Input: dimensioned drawing with shaded views. Units: mm. Origin: part minimum x, y, z. A direction names the side the tool comes from. Coordinates: 2 decimals unless noted, no trailing zeros. Write each loop counter-clockwise with the first axis right and the second up, starting at its lowest first coordinate (ties: lowest second). Pieces come first, ordered by that corner, then holes. Notation, with made-up numbers: (63, -21.75) - (114, -21.75) arc R12 ccw to (114, -8.75) - close; hole circle Ø5 at (22, 84). An arc over 180 degrees is marked (long way). One line per question, with ' | ' between items.
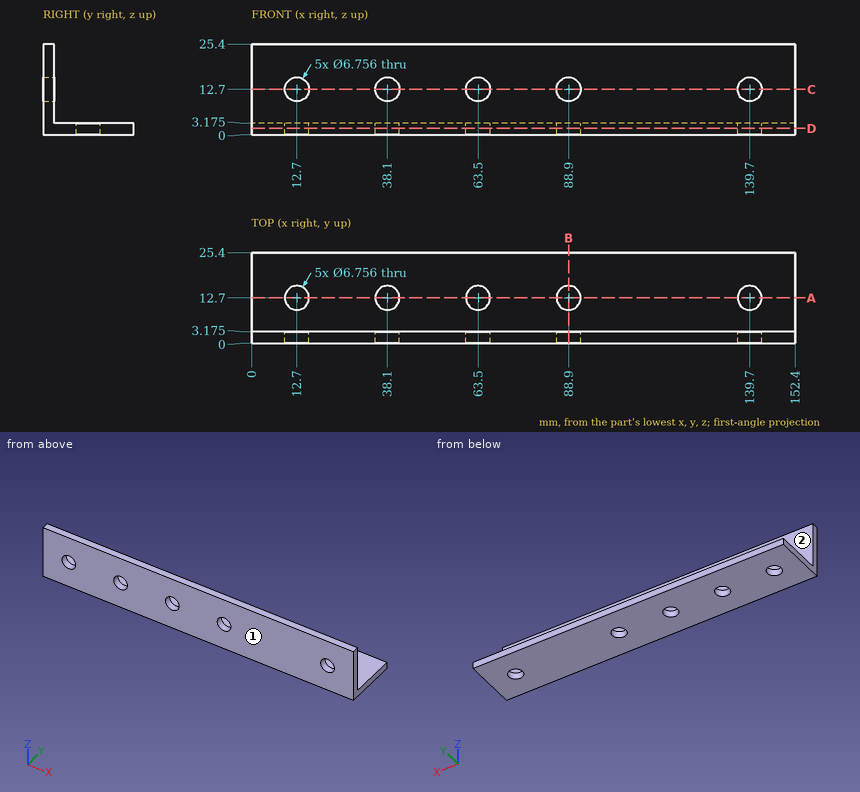
Item 1: Cut plane D-D on z = 1.75. Return loops of the section in (x, y).
Check sheet entries:
outline: (0, 0) - (152.4, 0) - (152.4, 25.4) - (0, 25.4) - close; hole circle Ø6.76 at (12.7, 12.7); hole circle Ø6.76 at (38.1, 12.7); hole circle Ø6.76 at (63.5, 12.7); hole circle Ø6.76 at (88.9, 12.7); hole circle Ø6.76 at (139.7, 12.7)
Item 2: Cut plane B-B on x = 88.9. Return loops of the section in (y, z) (1 decimal), and give its area (3 significant figures).
Check sheet entries:
outline: (0, 0) - (9.3, 0) - (9.3, 3.2) - (3.2, 3.2) - (3.2, 9.3) - (0, 9.3) - close; (0, 16.1) - (3.2, 16.1) - (3.2, 25.4) - (0, 25.4) - close; (16.1, 0) - (25.4, 0) - (25.4, 3.2) - (16.1, 3.2) - close | area: 108 mm²
Item 3: Cut plane A-A on y = 12.7. Return loops of the section in (x, z) (1 decimal).
Check sheet entries:
outline: (0, 0) - (9.3, 0) - (9.3, 3.2) - (0, 3.2) - close; (16.1, 0) - (34.7, 0) - (34.7, 3.2) - (16.1, 3.2) - close; (41.5, 0) - (60.1, 0) - (60.1, 3.2) - (41.5, 3.2) - close; (66.9, 0) - (85.5, 0) - (85.5, 3.2) - (66.9, 3.2) - close; (92.3, 0) - (136.3, 0) - (136.3, 3.2) - (92.3, 3.2) - close; (143.1, 0) - (152.4, 0) - (152.4, 3.2) - (143.1, 3.2) - close
Item 4: Ray query, line 1 along Z through (x, y) = (139.7, 0.9); line 2 along Y through (x, z) = (126.5, 21.5) (1 decimal). Return the intervals inside material, ascending. Write a range as [from, to].
Check sheet entries:
line 1: [0, 9.32], [16.08, 25.4] | line 2: [0, 3.2]
Item 5: Pin query (flat end, axial travel): pin 1 Ø11 at (x, z) = (12.7, 12.7) entering from +Y (3 decimals); pin 2 Ø3 at (x, y) = (79.5, 12.5) entering from +Z (3 decimals). Return the tip coordinate at first contact, or that it passes through.
Check sheet entries:
pin 1: y = 3.175 | pin 2: z = 3.175
Item 6: Access query for the marked faces 1 and 2. Directions: +Z, -Z, +X, -X, +Y, -Y. A direction counts if a zero-diameter tool reaches every point of the face in a straight line with its end or side. Return the directions, or none.
Check sheet entries:
face 1: +Z, -Z, +X, -X, -Y | face 2: +Z, +X, -X, +Y
